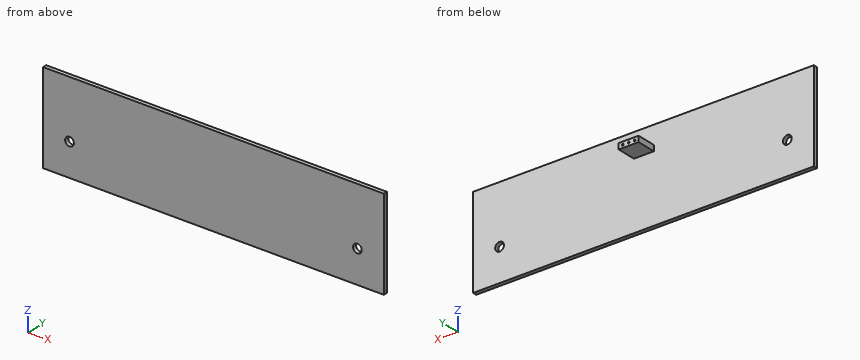
from build123d import *

# Parameters (mm, degrees)
ESQUISSE1_W             = 143.51
ESQUISSE1_H             = 38.1
BOSS_EXTRU_1_DEPTH      = 1.651
ESQUISSE2_R             = 1.8415
ENL_V_MAT_EXTRU_1_DEPTH = 75.259062248
ESQUISSE3_W             = 8.382
ESQUISSE3_H             = 2.413
BOSS_EXTRU_2_DEPTH      = 8.1788
ESQUISSE4_W             = 0.635
ESQUISSE4_H             = 0.635
ENL_V_MAT_EXTRU_2_DEPTH = 5.08


with BuildPart() as part:
    # Esquisse1 → Boss.-Extru.1 (new body)
    with BuildSketch(Plane(origin=(0, 0, 0), x_dir=(1, 0, 0), z_dir=(0, 1, 0))):
        Rectangle(ESQUISSE1_W, ESQUISSE1_H)
    extrude(amount=BOSS_EXTRU_1_DEPTH)

    # Esquisse2 → Enlèv. mat.-Extru.1 (cut, through all)
    with BuildSketch(Plane(origin=(0, 1.651, 0), x_dir=(1, 0, 0), z_dir=(0, 1, 0))):
        with Locations(Location((60.579, 5.334, 0), (0, 0, 270))):
            Circle(ESQUISSE2_R)
        with Locations(Location((-60.579, 5.334, 0), (0, 0, 270))):
            Circle(ESQUISSE2_R)
    extrude(amount=-ENL_V_MAT_EXTRU_1_DEPTH, mode=Mode.SUBTRACT)

    # Esquisse3 → Boss.-Extru.2 (add)
    with BuildSketch(Plane(origin=(0, 1.651, 0), x_dir=(1, 0, 0), z_dir=(0, 1, 0))):
        with Locations((-0.154698586, -10.2235)):
            Rectangle(ESQUISSE3_W, ESQUISSE3_H)
    extrude(amount=BOSS_EXTRU_2_DEPTH)

    # Esquisse4 → Enlèv. mat.-Extru.2 (cut)
    with BuildSketch(Plane(origin=(0, 9.8298, 0), x_dir=(1, 0, 0), z_dir=(0, 1, 0))):
        with Locations((-0.154698586, -10.2235)):
            Rectangle(ESQUISSE4_W, ESQUISSE4_H)
        with Locations((-2.694698586, -10.2235)):
            Rectangle(ESQUISSE4_W, ESQUISSE4_H)
        with Locations((2.385301414, -10.2235)):
            Rectangle(ESQUISSE4_W, ESQUISSE4_H)
    extrude(amount=-ENL_V_MAT_EXTRU_2_DEPTH, mode=Mode.SUBTRACT)


solid = part.part
Part model, mm, in its own coordinate system. Coordinates: 2 decimals unless noted, no trailing zeros. Order: outer loops, then holes, each group sorted by start corner. A loop starts at its lowest first (then second) coordinate and runs counter-clockwise, first axis right, second up. Notation, with made-up numbers: M 55,55.5 L 72,55.5 A18 ccw 72,89.5 Z; hole C -35,31 d11. An arc over 180 degrees is marked long. Use a Markdown table: item, result.
(1) Cut at A-A on y = 7.25. Write the cut outline in (x, z).
A:
| item | result |
|---|---|
| outline | M -4.35,9.02 L 4.04,9.02 L 4.04,11.43 L -4.35,11.43 Z; hole M -3.01,9.91 L -2.38,9.91 L -2.38,10.54 L -3.01,10.54 Z; hole M -0.47,9.91 L 0.16,9.91 L 0.16,10.54 L -0.47,10.54 Z; hole M 2.07,9.91 L 2.7,9.91 L 2.7,10.54 L 2.07,10.54 Z |
(2) Probe L1, parallel to X at y = 0.5, z = -5 (3 decimals); L2, parallel to Y at x = -32, z = 11.5. List the from-to ranges inside material, lowest first.
A:
| item | result |
|---|---|
| L1 | x = -71.755 to -62.39, -58.768 to 58.768, 62.39 to 71.755 |
| L2 | y = 0 to 1.65 |
(3) Cut at B-B on x = -8.5. Write the cut outline in (y, z), then the cut area to 3 significant figures.
A:
| item | result |
|---|---|
| outline | M 0,-19.05 L 1.65,-19.05 L 1.65,19.05 L 0,19.05 Z |
| area | 62.9 mm^2 |
(4) Flat gauge pins, fed straight in: pin 1 (0.5 mm diameter, centred on y = 7.5, z = 10, fed in from +X); pin 2 (0.7 mm diameter, centred on y = 6.5, z = 10, fed in from -X); pin 3 (3.5 mm diameter, centred on x = 60.579, z = -5.334, fed in from -Y); pin 4 (0.5 mm diameter, centred on x = 0, y = 8.5, fed in from -Z). Where does each tip first touch, or does it go through?
A:
| item | result |
|---|---|
| pin 1 | stops at x = 4.04 |
| pin 2 | stops at x = -4.35 |
| pin 3 | passes through |
| pin 4 | stops at z = 9.02 |
(5) Cut at C-C on z = 2.5. Write the cut outline in (x, y) (3 decimals), then the cut area to 3 significant figures.
A:
| item | result |
|---|---|
| outline | M -71.755,0 L 71.755,0 L 71.755,1.651 L -71.755,1.651 Z |
| area | 237 mm^2 |
